Here's how the part is built. I have some questions about the finished solid (model axes, mm). Face numbers are marked on the shaded views. A direction names the side the tool comes from. Round coordinates to 2 decimals unless told otherwise and drop trailing zeros. Loops run counter-clockwise (first coordinate to the right, second up) from the corner with the lowest first, then second, coordinate; pieces in that order, holes last. Notation, with made-up numbers: M -18,60 L 27,60 A20 ccw 27,69 Z; hole C 30.25,62.25 d2. An arc over 180 degrees is marked long. Use a Markdown table: item, result.
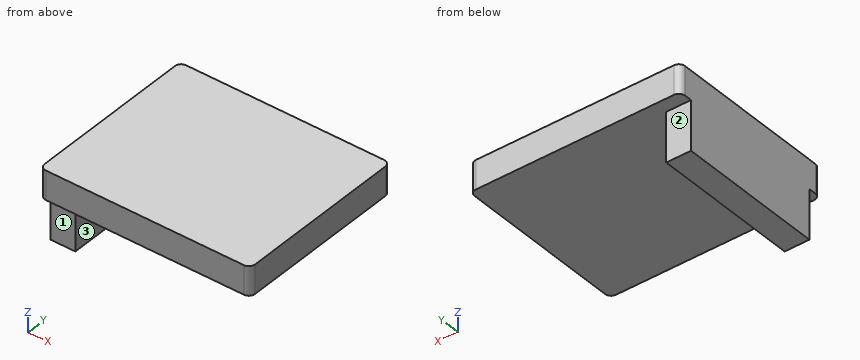
Autodesk Inventor part; units mm, degrees
ref_plane "YZ Plane" through (0, 0, 0) normal (1, 0, 0) x (0, 1, 0)
ref_plane "XZ Plane" through (0, 0, 0) normal (0, 1, 0) x (-1, 0, 0)
ref_plane "XY Plane" through (0, 0, 0) normal (0, 0, 1) x (1, 0, 0)
sketch "スケッチ1" plane through (0, 0, 0) normal (0, 0, 1) x (1, 0, 0)
  line L0 (-85, -71) -> (85, -71)
  line L1 (85, -71) -> (85, 71)
  line L2 (85, 71) -> (-85, 71)
  line L3 (-85, 71) -> (-85, -71)
  line L4 (-85, -71) -> (85, 71) construction
  line L5 (85, -71) -> (-85, 71) construction
  point P0 (0, 0)
  dimension "d0" = 170
  dimension "d1" = 142
extrude "押し出し1" add sketch "スケッチ1" along normal blind 23.35
fillet "フィレット1" radius 5 4 edges at (-85, 71, 11.675) (-85, -71, 11.675) (85, 71, 11.675) (85, -71, 11.675)
sketch "スケッチ2" plane through (0, 0, 0) normal (0, 0, 1) x (1, 0, 0)
  arc A0 (80, -71) -> (85, -66) centre (80, -66) ccw
  line L0 (85, -66) -> (85, 66)
  arc A1 (85, 66) -> (80, 71) centre (80, 66) ccw
  line L1 (80, 71) -> (-80, 71)
  arc A2 (-80, 71) -> (-85, 66) centre (-80, 66) ccw
  line L2 (-85, 66) -> (-85, -66)
  arc A3 (-85, -66) -> (-80, -71) centre (-80, -66) ccw
  line L3 (-80, -71) -> (80, -71)
  line L4 (-60, 51) -> (60, 51)
  line L5 (60, 51) -> (60, 71)
  line L6 (60, 71) -> (-60, 71)
  line L7 (-60, 71) -> (-60, 51)
  line L8 (-60, 51) -> (60, 71) construction
  line L9 (60, 51) -> (-60, 71) construction
  line L10 (80, 71) -> (-80, 71)
  line L11 (-20, 71) -> (-20, 51)
  line L12 (20, 51) -> (20, 71)
  line L13 (-65, 60) -> (-85, 60)
  line L14 (-85, 60) -> (-85, -60)
  line L15 (-85, -60) -> (-65, -60)
  line L16 (-65, -60) -> (-65, 60)
  line L17 (-65, 60) -> (-85, -60) construction
  line L18 (-85, 60) -> (-65, -60) construction
  point P0 (0, 0)
  point P1 (0, 61)
  point P2 (0, 61)
  point P3 (-75, 0)
  point P4 (-75, 0)
  dimension "d5" = 120
  dimension "d6" = 20
  dimension "d9" = 40
  dimension "d10" = 40
  dimension "d11" = 120
  dimension "d12" = 20
extrude "押し出し2" add sketch "スケッチ2" against normal blind 40 contours L2 L13 L16 L15
properties part number "base_link"
1. Imagine slicing it at B-B, the plane x = -61. Write out the boundary of the cut face in (y, z), then the cut area to 3 significant figures.
Answer sheet:
| item | result |
|---|---|
| outline | M -71,0 L 71,0 L 71,23.35 L -71,23.35 Z |
| area | 3,320 mm2 |
2. Which directions (+Z, -Z, +X, -X, +Y, -Y) give clear straight access to the entire face, cutting with the end or side of a thin tool? Please do the marked faces 1, 2 and 3.
Answer sheet:
| item | result |
|---|---|
| face 1 | -Z, +X, -X, -Y |
| face 2 | -Z, +X, -X, +Y |
| face 3 | -Z, +X, +Y, -Y |
3. Imagine slicing it at A-A, the plane y = 47. Write out the boundary of the cut face in (x, z).
Answer sheet:
| item | result |
|---|---|
| outline | M -85,-40 L -65,-40 L -65,0 L 85,0 L 85,23.35 L -85,23.35 Z |
4. For pin 1 Ø10 at (x, y) = (-26.5, -26) entering from -Z; pin 2 Ø20 at (y, z) = (19, -13.5) entering from +X; pin 3 Ø16 at (x, z) = (-73, -28) entering from +Y, each with a flat end and sliding along its axis, tell me the tip position at first contact or that it passes through.
Answer sheet:
| item | result |
|---|---|
| pin 1 | z = 0 |
| pin 2 | x = -65 |
| pin 3 | y = 60 |
5. Imagine slicing it at C-C, the plane z = -35. Write out the boundary of the cut face in (x, y), then the cut area to 3 significant figures.
Answer sheet:
| item | result |
|---|---|
| outline | M -85,-60 L -65,-60 L -65,60 L -85,60 Z |
| area | 2,400 mm2 |
6. I need wall thicknesses on probe 1 along X at (y, z) = (55, -12); probe 2 along Z at (x, y) = (9, -10). Which ranges of each line are inside material? Lowest first, please. Write a range as from..to.
Answer sheet:
| item | result |
|---|---|
| probe 1 | -85..-65 |
| probe 2 | 0..23.35 |
